from build123d import *

# Parameters (mm, degrees)
SKETCH1_W                   = 127.89
SKETCH1_H                   = 85.6
MAIN_PLATE_DEPTH            = 20.02
WELLS_LSP_R                 = 7.81
WELLS_DEPTH_DEPTH           = 17.14
SKETCH7_W                   = 127.89
SKETCH7_H                   = 85.6
SKETCH7_W_2                 = 124.89
SKETCH7_H_2                 = 82.6
FLANGE_DEPTH                = 6.57
STYLE_3_DEPTH               = 6.57
THICKNESS_SHELLING_T        = -0.32
ADDT_L_START                = 0.95
WELL_ELEVATOR_R             = 7.81
ADDT_L_WELL_ELEVATION_DEPTH = 0.95
FLANGE_STYLE_FILLETS_R      = 3
PLATE_EDGE_FILLETS_R        = 3


with BuildPart() as part:
    # Sketch1 → Main Plate (new body)
    with BuildSketch(Plane(origin=(0, 0, 0), x_dir=(1, 0, 0), z_dir=(0, 1, 0))):
        Rectangle(SKETCH1_W, SKETCH1_H)
    extrude(amount=MAIN_PLATE_DEPTH)

    # Wells_LSP → Wells Depth (cut)
    with BuildSketch(Plane(origin=(0, 20.02, 0), x_dir=(1, 0, 0), z_dir=(0, 1, 0))):
        with Locations(Location((-46.425, 28.96, 0), (0, 0, 270))):
            Circle(WELLS_LSP_R)
        with Locations(Location((-27.125, 28.96, 0), (0, 0, 270))):
            Circle(WELLS_LSP_R)
        with Locations(Location((-7.825, 28.96, 0), (0, 0, 270))):
            Circle(WELLS_LSP_R)
        with Locations(Location((11.475, 28.96, 0), (0, 0, 270))):
            Circle(WELLS_LSP_R)
        with Locations(Location((30.775, 28.96, 0), (0, 0, 270))):
            Circle(WELLS_LSP_R)
        with Locations(Location((50.075, 28.96, 0), (0, 0, 270))):
            Circle(WELLS_LSP_R)
        with Locations(Location((-27.125, 9.66, 0), (0, 0, 270))):
            Circle(WELLS_LSP_R)
        with Locations(Location((-7.825, 9.66, 0), (0, 0, 270))):
            Circle(WELLS_LSP_R)
        with Locations(Location((11.475, 9.66, 0), (0, 0, 270))):
            Circle(WELLS_LSP_R)
        with Locations(Location((30.775, 9.66, 0), (0, 0, 270))):
            Circle(WELLS_LSP_R)
        with Locations(Location((50.075, 9.66, 0), (0, 0, 270))):
            Circle(WELLS_LSP_R)
        with Locations(Location((-27.125, -9.64, 0), (0, 0, 270))):
            Circle(WELLS_LSP_R)
        with Locations(Location((-7.825, -9.64, 0), (0, 0, 270))):
            Circle(WELLS_LSP_R)
        with Locations(Location((11.475, -9.64, 0), (0, 0, 270))):
            Circle(WELLS_LSP_R)
        with Locations(Location((30.775, -9.64, 0), (0, 0, 270))):
            Circle(WELLS_LSP_R)
        with Locations(Location((50.075, -9.64, 0), (0, 0, 270))):
            Circle(WELLS_LSP_R)
        with Locations(Location((-27.125, -28.94, 0), (0, 0, 270))):
            Circle(WELLS_LSP_R)
        with Locations(Location((-7.825, -28.94, 0), (0, 0, 270))):
            Circle(WELLS_LSP_R)
        with Locations(Location((11.475, -28.94, 0), (0, 0, 270))):
            Circle(WELLS_LSP_R)
        with Locations(Location((30.775, -28.94, 0), (0, 0, 270))):
            Circle(WELLS_LSP_R)
        with Locations(Location((50.075, -28.94, 0), (0, 0, 270))):
            Circle(WELLS_LSP_R)
        with Locations(Location((-46.425, 9.66, 0), (0, 0, 270))):
            Circle(WELLS_LSP_R)
        with Locations(Location((-46.425, -9.64, 0), (0, 0, 270))):
            Circle(WELLS_LSP_R)
        with Locations(Location((-46.425, -28.94, 0), (0, 0, 270))):
            Circle(WELLS_LSP_R)
    extrude(amount=-WELLS_DEPTH_DEPTH, mode=Mode.SUBTRACT)

    # Sketch7 → Flange (cut)
    with BuildSketch(Plane(origin=(0, 20.02, 0), x_dir=(1, 0, 0), z_dir=(0, 1, 0))):
        Rectangle(SKETCH7_W, SKETCH7_H)
        Rectangle(SKETCH7_W_2, SKETCH7_H_2, mode=Mode.SUBTRACT)
    extrude(amount=-FLANGE_DEPTH, mode=Mode.SUBTRACT)

    # Style Sketch → Style <3 (cut)
    with BuildSketch(Plane(origin=(0, 20.02, 0), x_dir=(1, 0, 0), z_dir=(0, 1, 0))):
        Polygon((-62.445, 41.3), (-52.445, 41.3), (-62.445, 31.3), align=None)
        Polygon((-62.445, -41.3), (-52.445, -41.3), (-62.445, -31.3), align=None)
    extrude(amount=-STYLE_3_DEPTH, mode=Mode.SUBTRACT)

    # Thickness Shelling
    thickness_shelling_openings = [part.faces().sort_by_distance(p)[0] for p in [
        (0, 0, 0),
    ]]
    offset(amount=THICKNESS_SHELLING_T, openings=thickness_shelling_openings, kind=Kind.INTERSECTION)

    # Well Elevator → Addt'l Well Elevation (add)
    with BuildSketch(Plane(origin=(0, 2.88, 0), x_dir=(1, 0, 0), z_dir=(0, 1, 0)).offset(ADDT_L_START)):
        with Locations(Location((-46.425, 28.96, 0), (0, 0, 270))):
            Circle(WELL_ELEVATOR_R)
        with Locations(Location((-27.125, 28.96, 0), (0, 0, 270))):
            Circle(WELL_ELEVATOR_R)
        with Locations(Location((-7.825, 28.96, 0), (0, 0, 270))):
            Circle(WELL_ELEVATOR_R)
        with Locations(Location((11.475, 28.96, 0), (0, 0, 270))):
            Circle(WELL_ELEVATOR_R)
        with Locations(Location((30.775, 28.96, 0), (0, 0, 270))):
            Circle(WELL_ELEVATOR_R)
        with Locations(Location((50.075, 28.96, 0), (0, 0, 270))):
            Circle(WELL_ELEVATOR_R)
        with Locations(Location((-27.125, 9.66, 0), (0, 0, 270))):
            Circle(WELL_ELEVATOR_R)
        with Locations(Location((-7.825, 9.66, 0), (0, 0, 270))):
            Circle(WELL_ELEVATOR_R)
        with Locations(Location((11.475, 9.66, 0), (0, 0, 270))):
            Circle(WELL_ELEVATOR_R)
        with Locations(Location((30.775, 9.66, 0), (0, 0, 270))):
            Circle(WELL_ELEVATOR_R)
        with Locations(Location((50.075, 9.66, 0), (0, 0, 270))):
            Circle(WELL_ELEVATOR_R)
        with Locations(Location((-27.125, -9.64, 0), (0, 0, 270))):
            Circle(WELL_ELEVATOR_R)
        with Locations(Location((-7.825, -9.64, 0), (0, 0, 270))):
            Circle(WELL_ELEVATOR_R)
        with Locations(Location((11.475, -9.64, 0), (0, 0, 270))):
            Circle(WELL_ELEVATOR_R)
        with Locations(Location((30.775, -9.64, 0), (0, 0, 270))):
            Circle(WELL_ELEVATOR_R)
        with Locations(Location((50.075, -9.64, 0), (0, 0, 270))):
            Circle(WELL_ELEVATOR_R)
        with Locations(Location((-27.125, -28.94, 0), (0, 0, 270))):
            Circle(WELL_ELEVATOR_R)
        with Locations(Location((-7.825, -28.94, 0), (0, 0, 270))):
            Circle(WELL_ELEVATOR_R)
        with Locations(Location((11.475, -28.94, 0), (0, 0, 270))):
            Circle(WELL_ELEVATOR_R)
        with Locations(Location((30.775, -28.94, 0), (0, 0, 270))):
            Circle(WELL_ELEVATOR_R)
        with Locations(Location((50.075, -28.94, 0), (0, 0, 270))):
            Circle(WELL_ELEVATOR_R)
        with Locations(Location((-46.425, 9.66, 0), (0, 0, 270))):
            Circle(WELL_ELEVATOR_R)
        with Locations(Location((-46.425, -9.64, 0), (0, 0, 270))):
            Circle(WELL_ELEVATOR_R)
        with Locations(Location((-46.425, -28.94, 0), (0, 0, 270))):
            Circle(WELL_ELEVATOR_R)
    extrude(amount=-ADDT_L_WELL_ELEVATION_DEPTH)

    # Flange/Style Fillets
    flange_style_fillets_edges = [part.edges().sort_by_distance(p)[0] for p in [
        (62.445, 16.735, 41.3),
        (62.445, 16.735, -41.3),
        (-62.445, 16.735, -31.3),
        (-52.445, 16.735, -41.3),
        (-62.445, 16.735, 31.3),
        (-52.445, 16.735, 41.3),
        (62.125, 16.415, -40.98),
        (62.125, 16.415, 40.98),
        (-62.125, 16.415, 31.16745166),
        (-52.31245166, 16.415, -40.98),
        (-62.125, 16.415, -31.16745166),
        (-52.31245166, 16.415, 40.98),
    ]]
    fillet(flange_style_fillets_edges, radius=FLANGE_STYLE_FILLETS_R)

    # Plate Edge Fillets
    plate_edge_fillets_edges = [part.edges().sort_by_distance(p)[0] for p in [
        (63.945, 6.725, 42.8),
        (-63.945, 6.725, 42.8),
        (-63.945, 6.725, -42.8),
        (63.945, 6.725, -42.8),
        (-63.625, 6.565, 42.48),
        (-63.625, 6.565, -42.48),
        (63.625, 6.565, -42.48),
        (63.625, 6.565, 42.48),
    ]]
    fillet(plate_edge_fillets_edges, radius=PLATE_EDGE_FILLETS_R)


solid = part.part
Design review of the part built by this model. Coordinates are the model's own, in mm. A direction names the side the tool comes from. Round coordinates to 2 decimals unless told otherwise and drop trailing zeros. Use one line per item in the form item = value. Start each with the question number.
Q1. Wall thickness on line 1 along Z through (x, y) = (24, 1.25); line 2 along Y through (x, z) = (-37, 17); line 3 along Y through (x, z) = (-45.5, -22): over which ranges is each line inside the solid? List them lowest first. Write a range as [from, to].
Q2. Draft analysis for pull direction Z (two halves, no side actions). For faces 1 (the face through (-63.09, 6.82, 41.9)), 2 (the face through (-27, 2.56, 29)), 3 (the face through (3, 17, -41.3)), state which applies: +Z half, -Z half, draft (parallel to the pull), parting line (faces both ways), or undercut.
Q3. We need section A-A on y = 16.75. State how many separate pieces and enclosed holes the cut face has, then the cut area to 3 significant figures.
Q4. Machinability: for faces 4 (the face through (-10.94, 11.25, -21.45)), 5 (the face through (-63.09, 6.82, -41.9)), 6 (the face through (-27, 3.83, 10)), which of the approach directions +Z, -Z, +X, -X, +Y, -Y give a long, thin tool a straight path to every point of the face, cutting with its end or side? Answer none if there is none.
Q5. For pin 1 Ø4 at (x, z) = (-9, 9) entering from +Y; pin 2 Ø18 at (x, z) = (-46.425, -9.66) entering from -Y; pin 3 Ø2 at (y, z) = (17, -22.5) entering from +X (3 decimals), all flat-tipped, find the tip position at first contact; note any pin that passes through.
Calculated:
q1.line_1 = [-42.8, -42.48], [42.48, 42.8]
q1.line_2 = [19.7, 20.02]
q1.line_3 = [2.56, 3.83]
q2.face_1 = +Z half
q2.face_2 = undercut
q2.face_3 = -Z half
q3.separate_pieces = 25
q3.enclosed_holes = 25
q3.area = 513 mm²
q4.face_4 = -Y
q4.face_5 = -Z, -X, +Y, -Y
q4.face_6 = +Y
q5.pin_1 = 3.83
q5.pin_2 = 2.56
q5.pin_3 = 62.445
